The model under review builds one solid part; all positions refer to its coordinate system, in mm. Coordinates: 2 decimals unless noted, no trailing zeros. Write each loop counter-clockwise with the first axis right and the second up, starting at its lowest first coordinate (ties: lowest second). Pieces come first, ordered by that corner, then holes. Notation, with made-up numbers: M 48,-9.5 L 86,-9.5 A11 ccw 86,4.5 Z; hole C 82,-14 d5. An arc over 180 degrees is marked long. Answer as a JSON object with one key per item and string values.
```python
from build123d import *

# Parameters (mm, degrees)
F0_R     = 139.7
F0_R_2   = 122.5
F1_DEPTH = 6
F2_R     = 139.1
F2_R_2   = 122.5
F3_DEPTH = 3.59
F4_R     = 135.7
F4_R_2   = 122.5
F5_DEPTH = 36
F6_R     = 131
F6_R_2   = 122.5
F7_DEPTH = 2
F8_R     = 4


with BuildPart() as f1:
    # F0 (on Front) → F1 (new body)
    with BuildSketch(Plane.XZ):
        Circle(F0_R)
        Circle(F0_R_2, mode=Mode.SUBTRACT)
    extrude(amount=F1_DEPTH)

    # F2 (on face) → F3 (join)
    with BuildSketch(Plane.XZ.offset(6)):
        Circle(F2_R)
        Circle(F2_R_2, mode=Mode.SUBTRACT)
    extrude(amount=F3_DEPTH)

    # F4 (on face) → F5 (join)
    with BuildSketch(Plane(origin=(0, 0, 0), x_dir=(-1, 0, 0), z_dir=(0, 1, 0))):
        Circle(F4_R)
        Circle(F4_R_2, mode=Mode.SUBTRACT)
    extrude(amount=F5_DEPTH)

    # F6 (on face) → F7 (cut)
    with BuildSketch(Plane.XZ.offset(9.59)):
        Circle(F6_R)
        Circle(F6_R_2, mode=Mode.SUBTRACT)
    extrude(amount=-F7_DEPTH, mode=Mode.SUBTRACT)

    # F8
    f8_edges = [f1.edges().sort_by_distance(p)[0] for p in [
        (135.7, 36, 0),
    ]]
    fillet(f8_edges, radius=F8_R)


solid = f1.part
```
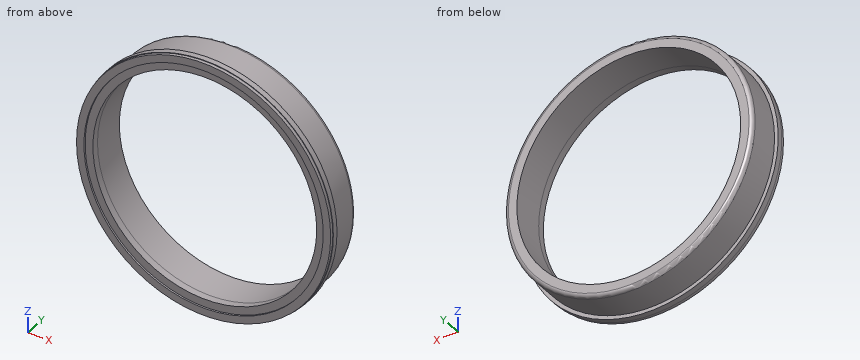
(1) Wall thickness on line 1 along Z through (x, y) = (0, -2.75); line 2 along Z through (x, y) = (0, -8); line 3 along X through (y, z) = (27, 72): over which ranges is each line inside the solid? List them lowest first. Write a range as from..to.
Results list:
{"line 1": "-139.7..-122.5, 122.5..139.7", "line 2": "-139.1..-131, 131..139.1", "line 3": "-115.02..-99.11, 99.11..115.02"}
(2) For pin 1 Ø10 at (y, z) = (16.5, -50) entering from +X; pin 2 Ø3 at (y, z) = (8.5, 67) entering from -X; pin 3 Ø4 at (y, z) = (30.5, 85) entering from +X, all flat-tipped, find the tip position at first contact; note any pin that passes through.
Results list:
{"pin 1": "x = 128.02", "pin 2": "x = -118.85", "pin 3": "x = 107.36"}
(3) Add section C-C on y = 23.5. Give the boundary of the cut face in (x, z).
Results list:
{"outline": "C 0,0 d271.4; hole C 0,0 d245"}
(4) Add section A-A on z = 0. Give the boundary of the cut face in (x, y).
Results list:
{"outline": "M -139.7,-6 L -139.1,-6 L -139.1,-9.59 L -131,-9.59 L -131,-7.59 L -122.5,-7.59 L -122.5,36 L -131.7,36 A4 ccw -135.7,32 L -135.7,0 L -139.7,0 Z; M 122.5,-7.59 L 131,-7.59 L 131,-9.59 L 139.1,-9.59 L 139.1,-6 L 139.7,-6 L 139.7,0 L 135.7,0 L 135.7,32 A4 ccw 131.7,36 L 122.5,36 Z"}
(5) Add section B-B on x = 0. Give the boundary of the cut face in (y, z), and give its area (3 significant figures).
Results list:
{"outline": "M -9.59,-139.1 L -6,-139.1 L -6,-139.7 L 0,-139.7 L 0,-135.7 L 32,-135.7 A4 ccw 36,-131.7 L 36,-122.5 L -7.59,-122.5 L -7.59,-131 L -9.59,-131 Z; M -9.59,131 L -7.59,131 L -7.59,122.5 L 36,122.5 L 36,131.7 A4 ccw 32,135.7 L 0,135.7 L 0,139.7 L -6,139.7 L -6,139.1 L -9.59,139.1 Z", "area": "1,240 mm²"}
